Drawing for the job (mm, zero at the part's lowest x, y, z). A direction names the side the tool comes from. Round coordinates to 2 decimals unless told otherwise and drop trailing zeros. Loops run counter-clockwise (first coordinate to the right, second up) from the corner with the lowest first, then second, coordinate; pieces in that order, holes last. Notation, with made-up numbers: M 61.25,64 L 91.25,64 A18 cw 91.25,86 Z; hole C -15.5,-24.75 d5. An arc over 180 degrees is marked long. Write each question's results on one line, items separated by ' | '.
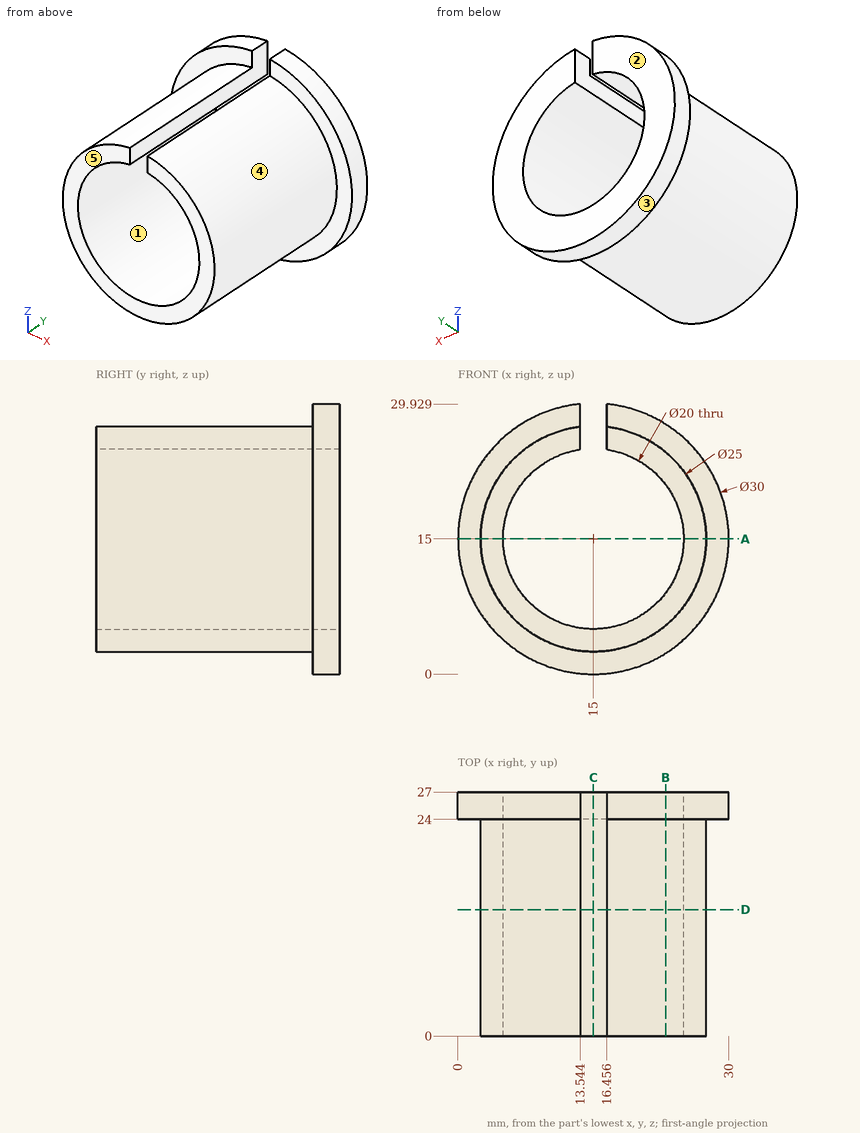
Item 1: Drop flat-ended pins along their axis: P1, Ø1, axis at y = 16.5, z = 8.5, coming from the +X side (1 decimal); P2, Ø5.5, axis at y = 17, z = 27, coming from the +X side; P3, Ø1, axis at x = 18.5, y = 13.5, coming from the +Z side (1 decimal); P4, Ø1.5, axis at x = 3.5, z = 3.5, coming from the -Y side. Give the stop position or say it passes through.
Filled sheet:
P1: x = 26 | P2: x = 23.41 | P3: z = 27.1 | P4: through
Item 2: Wall check: L1, parallel to X at y = 8.25, z = 15; L2, parallel to Z at x = 9, y = 9.75 (1 decimal); L3, parallel to X at y = 10.75, z = 6 (1 decimal). Give the ranges that are in metal, low to high.
Filled sheet:
L1: 2.5 to 5, 25 to 27.5 | L2: 4 to 7, 23 to 26 | L3: 6.3 to 10.6, 19.4 to 23.7
Item 3: Which spindle directions (+Z, -Z, +X, -X, +Y, -Y) get a long thin tool onto all of the face, cutting with end or side? Do the marked faces 4 and 5. Say none if no direction does.
Filled sheet:
face 4: -Y | face 5: +Z, -Z, +X, -X, -Y
Item 4: Band-saw the part on C-C on x = 15. Give the cut face in (y, z).
Filled sheet:
outline: M 0,2.5 L 24,2.5 L 24,0 L 27,0 L 27,5 L 0,5 Z
Item 5: Band-saw the part on D-D on y = 14. Give the cut face in (x, z) (1 decimal).
Filled sheet:
outline: M 13.5,24.9 L 13.5,27.4 A12.5 ccw long 16.5,27.4 L 16.5,24.9 A10 cw long Z
Item 6: Two-plate mould, pull along X, no slides. Class the marked faces 1, 2 and 3: +X half, -X half, draft (parallel to the pull), parting line (faces both ways), or undercut.
Filled sheet:
face 1: undercut | face 2: draft | face 3: parting line
Item 7: Band-saw the part on B-B on x = 23. Give the cut face in (y, z) (1 decimal), and give its area (3 significant figures).
Filled sheet:
outline: M 0,5.4 L 24,5.4 L 24,2.3 L 27,2.3 L 27,9 L 0,9 Z; M 0,21 L 27,21 L 27,27.7 L 24,27.7 L 24,24.6 L 0,24.6 Z | area: 213 mm^2
Item 8: Band-saw the part on A-A on z = 15. Give the cut face in (x, y), and give its area (3 significant figures).
Filled sheet:
outline: M 0,24 L 2.5,24 L 2.5,0 L 5,0 L 5,27 L 0,27 Z; M 25,0 L 27.5,0 L 27.5,24 L 30,24 L 30,27 L 25,27 Z | area: 150 mm^2
